Design review of the part shown in the three views and the two pictorial views. Dimensions are in mm from the part's minimum x, y and z. Round coordinates to 2 decimals unless told otherwise and drop trailing zeros. Order: outer loops, then holes, each group sorted by start corner. A loop starts at its lowest first (then second) coordinate and runs counter-clockwise, first axis right, second up.
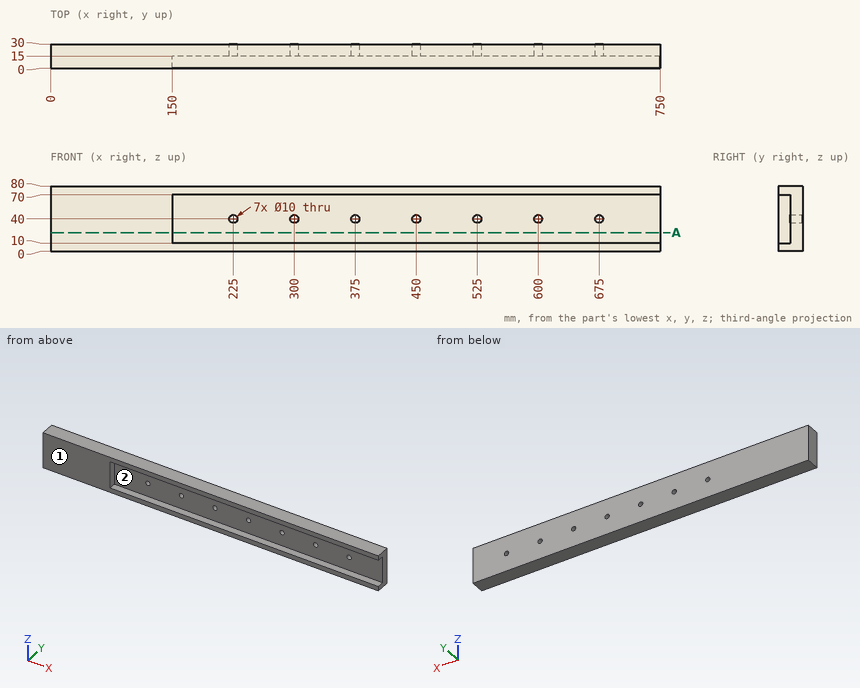
(1) Add section A-A on z = 23. Give the boundary of the cut face in (x, y), plus the area to 3 significant figures.
(2) Clearance check with flat-ended pins moving along their axes: P1, Ø13, axis at x = 300, z = 40, coming from the -Y side; P2, Ø4.5, axis at y = 8, z = 37.5, coming from the +X side. State where each tip first meets the part, or that it passes through.
(3) Wall thickness on L1, parallel to Z at x = 231, y = 8.5; L2, parallel to Z at x = 225, y = 19.75; L3, parallel to Y at x = 694.5, z = 61: over which ranges is each line inside the solid? List them lowest first.
(4) Draft analysis for pull direction Z (two halves, no side actions). For the marked faces 1 and 2, state which applies: pulls with the +Z half, pulls with the -Z half, needs draft (parallel to the pull), parting line crosses it, or undercut.
Here are the results:
1. outline: (0, 0) - (150, 0) - (150, 15) - (750, 15) - (750, 30) - (0, 30) - close
1. area: 13,500 mm2
2. P1: stops at y = 15
2. P2: stops at x = 150
3. L1: z = 0 to 10, 70 to 80
3. L2: z = 0 to 35, 45 to 80
3. L3: y = 15 to 30
4. face 1: needs draft
4. face 2: undercut
